For this review, take the finished solid that the model builds, in its own axes (mm). A direction names the side the tool comes from. Give positions to 0.01 mm unless a question says otherwise; leave off trailing zeros. Loops run counter-clockwise (first coordinate to the right, second up) from the corner with the lowest first, then second, coordinate; pieces in that order, holes last. Notation, with made-up numbers: (-37, -26.5) - (-27, -26.5) arc R21 cw to (-27, -22.5) - close; hole circle Ø7 at (52, 60). An arc over 180 degrees is marked (long way). Answer in a Markdown table with one row per item.
```python
from build123d import *

# Parameters (mm, degrees)
SALIENTE_EXTRUIR1_DEPTH = 180
CORTAR_EXTRUIR1_DEPTH   = 5
CROQUIS3_W              = 40
CROQUIS3_H              = 83
CORTAR_EXTRUIR2_DEPTH   = 5


with BuildPart() as part:
    # Croquis1 → Saliente-Extruir1 (new body)
    with BuildSketch(Plane(origin=(0, 0, 0), x_dir=(1, 0, 0), z_dir=(0, 1, 0))):
        Polygon((0, 0), (-50, 0), (-50, 5), (-5, 5), (-5, 50), (0, 50), align=None)
    extrude(amount=SALIENTE_EXTRUIR1_DEPTH)

    # Croquis2 → Cortar-Extruir1 (cut)
    with BuildSketch(Plane(origin=(0, 0, 0), x_dir=(0, 0, -1), z_dir=(1, 0, 0))):
        Polygon((50, 95), (16.666666667, 0), (50, 0), align=None)
    extrude(amount=-CORTAR_EXTRUIR1_DEPTH, mode=Mode.SUBTRACT)

    # Croquis3 → Cortar-Extruir2 (cut)
    with BuildSketch(Plane.XY):
        with Locations((-30, 138.5)):
            Rectangle(CROQUIS3_W, CROQUIS3_H)
    extrude(amount=-CORTAR_EXTRUIR2_DEPTH, mode=Mode.SUBTRACT)


solid = part.part
```
1. We need section C-C, the plane z = -11.5. Give the boundary of the cut face in (x, y).
Values:
| item | result |
|---|---|
| outline | (-5, 0) - (0, 0) - (0, 180) - (-5, 180) - close |
2. We need section D-D, the plane z = -45. Give the boundary of the cut face in (x, y), and give its area (3 significant figures).
Values:
| item | result |
|---|---|
| outline | (-5, 80.75) - (0, 80.75) - (0, 180) - (-5, 180) - close |
| area | 496 mm^2 |
3. Wall thickness on line 1 (X direction, y = 154.5, z = -28); line 2 (X direction, y = 161.5, z = -3): over which ranges is each line inside the solid? List them lowest first. Write a range as [from, to].
Values:
| item | result |
|---|---|
| line 1 | x = [-5, 0] |
| line 2 | x = [-10, 0] |
4. Clearance check with flat-ended pins moving along their axes: pin 1 (1.5 mm diameter, centred on y = 81.5, z = -21.5, fed in from -X); pin 2 (5.5 mm diameter, centred on y = 134.5, z = -1.5, fed in from -X); pin 3 (2.5 mm diameter, centred on x = -29.5, z = -1.5, fed in from +Y); pin 4 (8 mm diameter, centred on y = 42.5, z = -38.5, fed in from -X). State where each tip first meets the part, or that it passes through.
Values:
| item | result |
|---|---|
| pin 1 | stops at x = -5 |
| pin 2 | stops at x = -10 |
| pin 3 | stops at y = 97 |
| pin 4 | passes through |
5. We need section A-A, the plane x = -3. Give the boundary of the cut face in (y, z).
Values:
| item | result |
|---|---|
| outline | (0, -16.67) - (95, -50) - (180, -50) - (180, 0) - (0, 0) - close |
6. We need section B-B, the plane y = 136.5. Give the boundary of the cut face in (x, z), and give its area (3 significant figures).
Values:
| item | result |
|---|---|
| outline | (-10, -5) - (-5, -5) - (-5, -50) - (0, -50) - (0, 0) - (-10, 0) - close |
| area | 275 mm^2 |
7. For faces 1 (the face through (-28, 49, -5)), 2 (the face through (-30, 97, -2)), 3 (the face through (0, 109, -20)), list the 3-axis set-ups (+Z, -Z, +X, -X, +Y, -Y) from which the entire face can be reached by the end or side of a thin tool; tool diameter is ignored.
Values:
| item | result |
|---|---|
| face 1 | -Z, -X, +Y, -Y |
| face 2 | +Z, -Z, -X, +Y |
| face 3 | +Z, -Z, +X, +Y, -Y |
